Can you work these out from the model? Positions are in its coordinate system, mm. Face numbers are marked on the shaded views. A direction names the side the tool comes from. Round coordinates to 2 decimals unless told otherwise and drop trailing zeros. Loops run counter-clockwise (first coordinate to the right, second up) from the corner with the lowest first, then second, coordinate; pieces in that order, holes last. Notation, with made-up numbers: (41, 50) -> (73, 50) arc R22 ccw to (73, 74) -> close; hole circle Ø5 at (38.25, 88). An arc over 180 degrees is marked (long way). Write item = value, one per line.
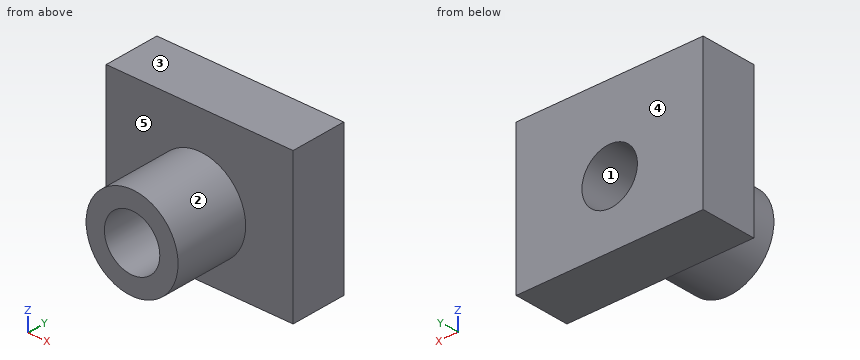
from build123d import *

# Parameters (mm, degrees)
F0_W     = 127
F0_H     = 101.6
F1_DEPTH = 38.1
F2_R     = 31.253705
F3_DEPTH = 50.8
F4_R     = 18.835615
F5_DEPTH = 88.901


with BuildPart() as f1:
    # F0 (on Front) → F1 (new body)
    with BuildSketch(Plane.XZ):
        Rectangle(F0_W, F0_H)
    extrude(amount=F1_DEPTH)

    # F2 (on face) → F3 (join)
    with BuildSketch(Plane.XZ.offset(38.1)):
        with Locations((0, -6.159689)):
            Circle(F2_R)
    extrude(amount=F3_DEPTH)

    # F4 (on face) → F5 (cut, through all)
    with BuildSketch(Plane.XZ.offset(88.9)):
        with Locations((0, -6.159689)):
            Circle(F4_R)
    extrude(amount=-F5_DEPTH, mode=Mode.SUBTRACT)


solid = f1.part
1. I'm going to push flat-ended pins straight in: pin 1 (1.5 mm diameter, centred on x = -24, y = -55, fed in from +Z); pin 2 (5 mm diameter, centred on y = -64.5, z = -26, fed in from +X); pin 3 (6 mm diameter, centred on x = 42.5, z = -26.5, fed in from +Y); pin 4 (2 mm diameter, centred on y = -80, z = 15, fed in from -X). Where does each tip first touch, or does it pass through?
Entries:
pin_1 = 14.73
pin_2 = 26
pin_3 = 0
pin_4 = -23.88
2. For the marked faces 4 and 5, which set-ups out of +Z, -Z, +X, -X, +Y, -Y let a thin tool reach every point of the face, with its end or its side?
Entries:
face_4 = +Z, -Z, +X, -X, +Y
face_5 = -Y
3. Suppose I cut it at B-B, the plane y = -27. List the corners of the cut face in (x, z) for me.
Entries:
outline = (-63.5, -50.8) -> (63.5, -50.8) -> (63.5, 50.8) -> (-63.5, 50.8) -> close; hole circle Ø37.67 at (0, -6.16)
4. Suppose I cut it at A-A, the plane x = 0. List the corners of the cut face in (y, z) for me.
Entries:
outline = (-88.9, -37.41) -> (-38.1, -37.41) -> (-38.1, -50.8) -> (0, -50.8) -> (0, -25) -> (-88.9, -25) -> close; (-88.9, 12.68) -> (0, 12.68) -> (0, 50.8) -> (-38.1, 50.8) -> (-38.1, 25.09) -> (-88.9, 25.09) -> close
5. We'd pull the mould along X, two halves only. Please class the marked faces 1, 2 and 3: released by +X, released by -X, zero draft, split by the parting line, or undercut.
Entries:
face_1 = undercut
face_2 = split by the parting line
face_3 = zero draft
6. I need wall thicknesses on line 1 (Z direction, x = 0, y = -25.5); line 2 (Z direction, x = 0, y = -63); line 3 (Y direction, x = 23.5, z = 21). Which ranges of each line are inside material? Lowest first, please. Write a range as [from, to].
Entries:
line_1 = [-50.8, -25], [12.68, 50.8]
line_2 = [-37.41, -25], [12.68, 25.09]
line_3 = [-38.1, 0]
7. Suppose I cut it at C-C, the plane z = -30. List the corners of the cut face in (x, y) for me.
Entries:
outline = (-63.5, -38.1) -> (-20.21, -38.1) -> (-20.21, -88.9) -> (20.21, -88.9) -> (20.21, -38.1) -> (63.5, -38.1) -> (63.5, 0) -> (-63.5, 0) -> close
8. Suppose I cut it at D-D, the plane x = -56. List the corners of the cut face in (y, z) for me.
Entries:
outline = (-38.1, -50.8) -> (0, -50.8) -> (0, 50.8) -> (-38.1, 50.8) -> close
